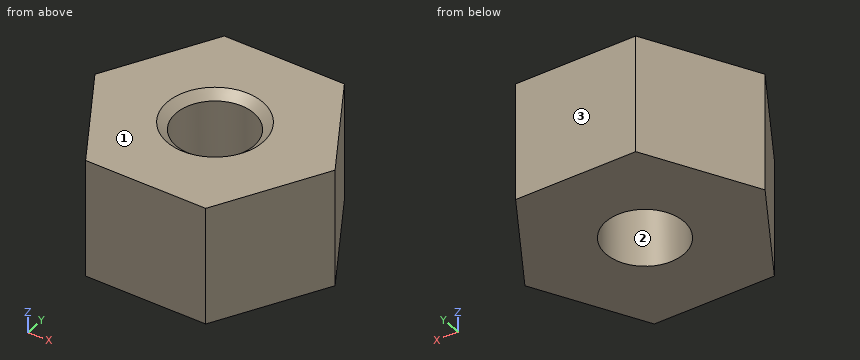
```python
from build123d import *

# Parameters (mm, degrees)
BOSS_EXTRUDE1_DEPTH             = 2.5
M4X0_7_TAPPED_HOLE1_D           = 3.3
M4X0_7_TAPPED_HOLE1_CSINK_D     = 4.05
M4X0_7_TAPPED_HOLE1_CSINK_ANGLE = 100


with BuildPart() as part:
    # Sketch1 → Boss-Extrude1 (new, symmetric)
    with BuildSketch(Plane.XY):
        Polygon((5, 0), (2.5, 4.330127019), (-2.5, 4.330127019), (-5, 0), (-2.5, -4.330127019), (2.5, -4.330127019), align=None)
    extrude(amount=BOSS_EXTRUDE1_DEPTH, both=True)

    # M4x0.7 Tapped Hole1 (through all)
    with Locations(Plane.XY.offset(2.5)):
        with Locations((0, 0)):
            CounterSinkHole(M4X0_7_TAPPED_HOLE1_D / 2, M4X0_7_TAPPED_HOLE1_CSINK_D / 2, counter_sink_angle=M4X0_7_TAPPED_HOLE1_CSINK_ANGLE)


solid = part.part
```
Build history of the part. All positions in model axes, mm. Face numbers are marked on the shaded views. Coordinates: 2 decimals unless noted, no trailing zeros. Order: outer loops, then holes, each group sorted by start corner. A loop starts at its lowest first (then second) coordinate and runs counter-clockwise, first axis right, second up. Notation, with made-up numbers: (47.5, 47.5) -> (81.5, 47.5) arc R25 cw to (81.5, 86.5) -> close; hole circle Ø6 at (28.5, 15.5). An arc over 180 degrees is marked (long way). Answer in a Markdown table with one row per item. Add a question column.
Q1. Wall check: line 1 along Y through (x, z) = (0, 0.75); line 2 along Y through (x, z) = (-1.25, -0.5); line 3 along X through (y, z) = (1.25, -2.2). Give the ranges that are in metal, low to high. Write a range as [from, to].
Q2. Mould opens along Y. For the marked faces 1, 2 and 3 say: +Y half, -Y half, draft (parallel to the pull), parting line (faces both ways), or undercut.
Q3. Band-saw the part on B-B, the plane z = -1.9. List the corners of the cut face in (x, y).
Q4. Band-saw the part on D-D, the plane x = -3.5. List the corners of the cut face in (y, z).
Q5. Drop a flat-ended pin along its axis: pin 1 (1.5 mm diameter, centred on y = 1, z = 0.5, fed in from -X). Give the stop position or say it passes through.
Q6. Band-saw the part on C-C, the plane y = -3.5. List the corners of the cut face in (x, z).
Q7. Band-saw the part on A-A, the plane x = 0. List the corners of the cut face in (y, z) (3 decimals), then the cut area to 3 significant figures.
Answers follow:
| question | item | result |
|---|---|---|
| 1 | line 1 | [-4.33, -1.65], [1.65, 4.33] |
| 1 | line 2 | [-4.33, -1.08], [1.08, 4.33] |
| 1 | line 3 | [-4.28, -1.08], [1.08, 4.28] |
| 2 | face 1 | draft |
| 2 | face 2 | undercut |
| 2 | face 3 | +Y half |
| 3 | outline | (-5, 0) -> (-2.5, -4.33) -> (2.5, -4.33) -> (5, 0) -> (2.5, 4.33) -> (-2.5, 4.33) -> close; hole circle Ø3.3 at (0, 0) |
| 4 | outline | (-2.6, -2.5) -> (2.6, -2.5) -> (2.6, 2.5) -> (-2.6, 2.5) -> close |
| 5 | pin 1 | x = -4.86 |
| 6 | outline | (-2.98, -2.5) -> (2.98, -2.5) -> (2.98, 2.5) -> (-2.98, 2.5) -> close |
| 7 | outline | (-4.33, -2.5) -> (-1.65, -2.5) -> (-1.65, 2.185) -> (-2.025, 2.5) -> (-4.33, 2.5) -> close; (1.65, -2.5) -> (4.33, -2.5) -> (4.33, 2.5) -> (2.025, 2.5) -> (1.65, 2.185) -> close |
| 7 | area | 26.7 mm^2 |
